Could you check a few things on this model? Use its own coordinates, in mm. A direction names the side the tool comes from. Coordinates: 2 decimals unless noted, no trailing zeros. Loops run counter-clockwise (first coordinate to the right, second up) from the corner with the lowest first, then second, coordinate; pieces in that order, holes last.
from build123d import *

# Parameters (mm, degrees)
F1_DEPTH = 38.1
F2_W     = 63.5
F2_H     = 31.75
F3_DEPTH = 19.05


with BuildPart() as f1:
    # F0 (on Front) → F1 (new body)
    with BuildSketch(Plane.XZ):
        Polygon((61.612287, -27.667911), (-1.887713, 4.082089), (-1.887713, -27.667911), align=None)
        Polygon((-1.887713, 4.082089), (-65.387713, 35.832089), (-65.387713, -27.667911), (-1.887713, -27.667911), align=None)
    extrude(amount=F1_DEPTH)

    # F2 (on Front) → F3 (join)
    with BuildSketch(Plane.XZ):
        with Locations((29.02056, -11.626451)):
            Rectangle(F2_W, F2_H)
    extrude(amount=F3_DEPTH)


solid = f1.part
(1) I need wall thicknesses on probe 1 along X at (y, z) = (-11, -18); probe 2 along X at (y, z) = (-30, 1); probe 3 along Z at (x, y) = (-36.5, -24.5). Which ranges of each line are inside material? Lowest first, please.
Answers:
probe 1: x = -65.39 to 60.77
probe 2: x = -65.39 to 4.28
probe 3: z = -27.67 to 21.39
(2) Imagine slicing it at B-B, the plane z = -19.5. Write out the boundary of the cut face in (x, y).
Answers:
outline: (-65.39, -38.1) - (45.28, -38.1) - (45.28, -19.05) - (60.77, -19.05) - (60.77, 0) - (-65.39, 0) - close
(3) Which directions (+Z, -Z, +X, -X, +Y, -Y) give clear straight access to the entire face, cutting with the end or side of a thin tool? Please do faces 1 (the face through (60.771, -9, -12)), 2 (the face through (-65.388, -19, 5)), 3 (the face through (43, -19.05, -4)).
Answers:
face 1: +Z, +X, +Y, -Y
face 2: +Z, -Z, -X, +Y, -Y
face 3: +Z, +X, -Y
(4) Imagine slicing it at D-D, the plane y = -21.5. Write out the boundary of the cut face in (x, z).
Answers:
outline: (-65.39, -27.67) - (61.61, -27.67) - (-65.39, 35.83) - close
(5) Imagine slicing it at C-C, the plane x = -27. Write out the boundary of the cut face in (y, z).
Answers:
outline: (-38.1, -27.67) - (0, -27.67) - (0, 16.64) - (-38.1, 16.64) - close
(6) For pin 1 (1.5 mm diameter, centred on x = -26.5, y = -18, fed in from +Z); pin 2 (6 mm diameter, centred on y = -30.5, z = 22, fed in from +X); pin 3 (9.5 mm diameter, centred on x = 34, y = -7.5, fed in from +Z); pin 4 (8 mm diameter, centred on x = 24, z = -6.5, fed in from +Y), each with a flat end and sliding along its axis, tell me the tip position at first contact or that it passes through.
Answers:
pin 1: stops at z = 16.76
pin 2: stops at x = -31.72
pin 3: stops at z = 4.25
pin 4: stops at y = 0
(7) Imagine slicing it at A-A, the plane y = -13. Write out the boundary of the cut face in (x, z), and give its area (3 significant figures).
Answers:
outline: (-65.39, -27.67) - (61.61, -27.67) - (60.77, -27.25) - (60.77, 4.25) - (-2.22, 4.25) - (-65.39, 35.83) - close
area: 5,020 mm2
